Design review of the part built by this model. Coordinates are the model's own, in mm. Face numbers are marked on the shaded views. A direction names the side the tool comes from. Coordinates: 2 decimals unless noted, no trailing zeros. Order: outer loops, then holes, each group sorted by start corner. A loop starts at its lowest first (then second) coordinate and runs counter-clockwise, first axis right, second up. Notation, with made-up numbers: (39, 29) - (94, 29) arc R25 cw to (94, 57) - close; hole circle Ø1 at (-28.5, 46.25). An arc over 180 degrees is marked (long way). Write item = value, one per line. Start each with the question number.
```python
from build123d import *

# Parameters (mm, degrees)
F0_W          = 20
F0_H          = 42
F0_R          = 2
F1_DEPTH      = 5
F0_W_2        = 8.5
F2_DEPTH      = 29
F2_DEPTH_BACK = 10
F0_R_2        = 1.5
F3_DEPTH      = 29
F4_DEPTH      = 24


# Not quite as in the source:
# - a feature names something its author has since deleted; it is built from what else it names


with BuildPart() as f1:
    # F0 (on Top) → F1 (new body)
    with BuildSketch(Plane.XY):
        with Locations((-2.5607131049, 21)):
            Rectangle(F0_W, F0_H)
        with Locations((-2.5607131049, 5.5)):
            Circle(F0_R, mode=Mode.SUBTRACT)
        with Locations((-2.5607131049, 36.5)):
            Circle(F0_R, mode=Mode.SUBTRACT)
    extrude(amount=F1_DEPTH)

    # F0 (on Top) → F2 (join, two sides)
    with BuildSketch(Plane.XY) as f2_sk:
        with Locations((11.6892868951, 21)):
            Rectangle(F0_W_2, F0_H)
    extrude(amount=F2_DEPTH)
    extrude(f2_sk.sketch, amount=-F2_DEPTH_BACK)

    # F0 (on Top) → F3 (join)
    with BuildSketch(Plane.XY):
        with BuildLine():
            ThreePointArc((28.9392868951, 13.4501655647), (25.9392868951, 21), (28.9392868951, 28.5498344353))
            Line((28.9392868951, 28.5498344353), (28.9392868951, 42))
            Line((28.9392868951, 42), (15.9392868951, 42))
            Line((15.9392868951, 42), (15.9392868951, 0))
            Line((15.9392868951, 0), (28.9392868951, 0))
            Line((28.9392868951, 0), (28.9392868951, 13.4501655647))
        make_face()
        with Locations((21.4392868951, 5.5)):
            Circle(F0_R_2, mode=Mode.SUBTRACT)
        with Locations((21.4392868951, 36.5)):
            Circle(F0_R_2, mode=Mode.SUBTRACT)
    extrude(amount=F3_DEPTH)

    # F0 (on Top) → F4 (cut)
    with BuildSketch(Plane.XY):
        with BuildLine():
            ThreePointArc((28.9392868951, 13.4501655647), (25.9392868951, 21), (28.9392868951, 28.5498344353))
            Line((28.9392868951, 28.5498344353), (28.9392868951, 42))
            Line((28.9392868951, 42), (15.9392868951, 42))
            Line((15.9392868951, 42), (15.9392868951, 0))
            Line((15.9392868951, 0), (28.9392868951, 0))
            Line((28.9392868951, 0), (28.9392868951, 13.4501655647))
        make_face()
        with Locations((21.4392868951, 5.5)):
            Circle(F0_R_2, mode=Mode.SUBTRACT)
        with Locations((21.4392868951, 36.5)):
            Circle(F0_R_2, mode=Mode.SUBTRACT)
    extrude(amount=F4_DEPTH, mode=Mode.SUBTRACT)


solid = f1.part
```
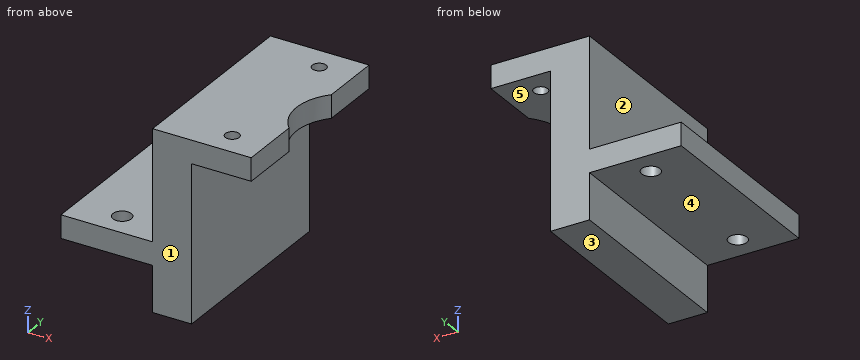
Item 1: Add section B-B on z = 1. Give the boundary of the cut face in (x, y).
Item 2: For P1, Ø10, axis at y = 18, z = 9.5, coming from the +X side; P2, Ø7, axis at y = 22.5, z = 18, coming from the -X side; P3, Ø4.5, axis at x = -2.56, y = 36.5, coming from the +Z side, all flat-tipped, find the tip position at first contact; note any pin that passes through.
Item 3: Add section D-D on x = 3. Give the boundary of the cut face in (y, z), plus the area to 3 significant figures.
Item 4: Add section C-C on x = 21. Give the boundary of the cut face in (y, z).
Item 5: For the marked faces 1, 2, 3, 4 and 5, list the 3-axis set-ups (+Z, -Z, +X, -X, +Y, -Y) from which the entire face can be reached by the end or side of a thin tool; tool diameter is ignored.
Item 6: Add section A-A on y = 36.5. Give the boundary of the cut face in (x, z).
Item 7: For line 1 (Z direction, x = -7.5, y = 34.5); line 2 (X direction, y = 33, z = 7.5); line 3 (Z direction, x = 21, y = 24), list the stretches that pass through material, from the lowest coordinate up.
Worked out:
q1.outline = (-12.56, 0) - (15.94, 0) - (15.94, 42) - (-12.56, 42) - close; hole circle Ø4 at (-2.56, 5.5); hole circle Ø4 at (-2.56, 36.5)
q2.P1 = 15.94
q2.P2 = 7.44
q2.P3 = 5
q3.outline = (0, 0) - (42, 0) - (42, 5) - (0, 5) - close
q3.area = 210 mm2
q4.outline = (0, 24) - (4.07, 24) - (4.07, 29) - (0, 29) - close; (6.93, 24) - (35.07, 24) - (35.07, 29) - (6.93, 29) - close; (37.93, 24) - (42, 24) - (42, 29) - (37.93, 29) - close
q5.face_1 = +Z, -Z, +X, -X, -Y
q5.face_2 = +Z, -X, +Y, -Y
q5.face_3 = -Z, +X, -X, +Y, -Y
q5.face_4 = -Z, -X, +Y, -Y
q5.face_5 = -Z, +X, +Y, -Y
q6.outline = (-12.56, 0) - (-4.56, 0) - (-4.56, 5) - (-12.56, 5) - close; (-0.56, 0) - (7.44, 0) - (7.44, -10) - (15.94, -10) - (15.94, 24) - (19.94, 24) - (19.94, 29) - (7.44, 29) - (7.44, 5) - (-0.56, 5) - close; (22.94, 24) - (28.94, 24) - (28.94, 29) - (22.94, 29) - close
q7.line_1 = 0 to 5
q7.line_2 = 7.44 to 15.94
q7.line_3 = 24 to 29
